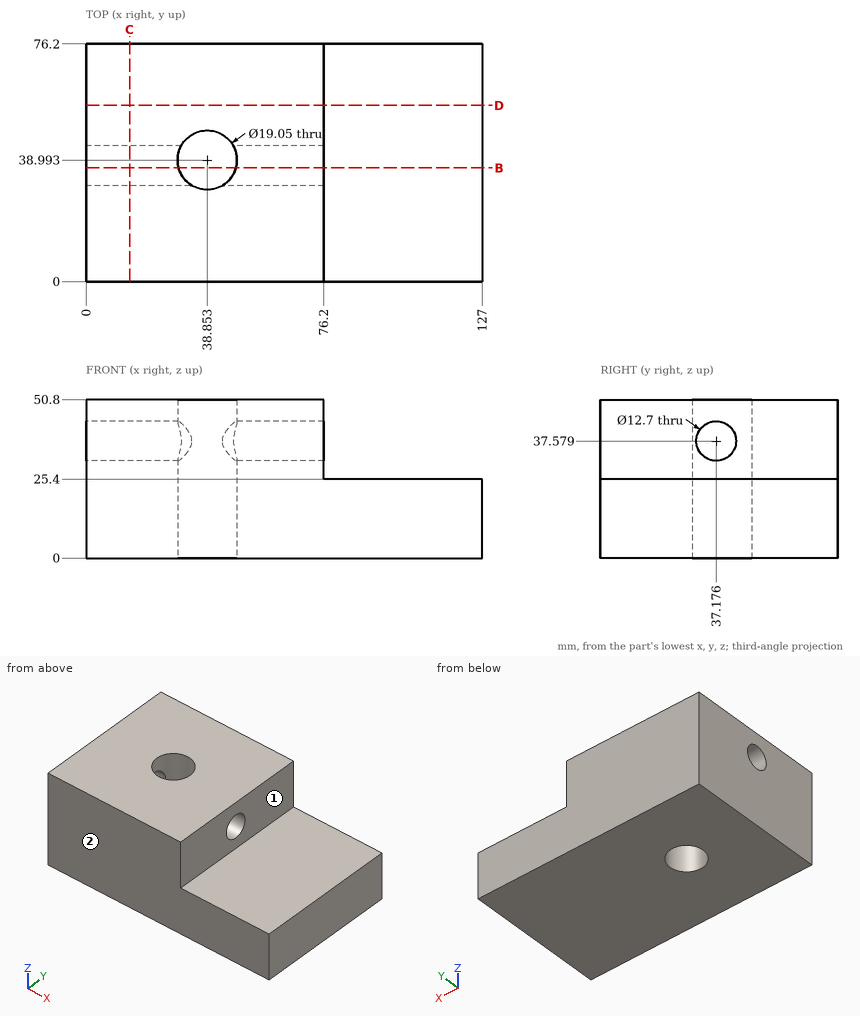
Check sheet for the drawn part. Datum: minimum x, y, z corner. Units: mm. A direction names the side the tool comes from. Coordinates: 2 decimals unless noted, no trailing zeros. Loops run counter-clockwise (first coordinate to the right, second up) from the corner with the lowest first, then second, coordinate; pieces in that order, holes last. Notation, with made-up numbers: (40.5, 66.5) -> (94.5, 66.5) arc R22 cw to (94.5, 80.5) -> close; hole circle Ø2 at (7, -28.75). An arc over 180 degrees is marked (long way). Answer in a Markdown table with one row per item.
1) Section check B-B (y = 36.5). Record the cut outline in (x, z) (1 decimal).
The answers:
| item | result |
|---|---|
| outline | (0, 0) -> (29.7, 0) -> (29.7, 31.3) -> (0, 31.3) -> close; (0, 43.9) -> (29.7, 43.9) -> (29.7, 50.8) -> (0, 50.8) -> close; (48, 0) -> (127, 0) -> (127, 25.4) -> (76.2, 25.4) -> (76.2, 31.3) -> (48, 31.3) -> close; (48, 43.9) -> (76.2, 43.9) -> (76.2, 50.8) -> (48, 50.8) -> close |
2) Section check D-D (y = 56.5). Record the cut outline in (x, z).
The answers:
| item | result |
|---|---|
| outline | (0, 0) -> (127, 0) -> (127, 25.4) -> (76.2, 25.4) -> (76.2, 50.8) -> (0, 50.8) -> close |
3) Depth check by flat-ended pin: P1, Ø10, axis at y = 37.18, z = 37.58, coming from the -X side; P2, Ø20.5, axis at y = 37.18, z = 37.58, coming from the +X side. Enter the tip coordinate at first touch or a pass-through.
The answers:
| item | result |
|---|---|
| P1 | passes through |
| P2 | stops at x = 76.2 |
4) Access from +Z, -Z, +X, -X, +Y, -Y to the whole of each face (thin tool, end or side, straight path). Record for the marked faces 1 and 2.
The answers:
| item | result |
|---|---|
| face 1 | +Z, +X, +Y, -Y |
| face 2 | +Z, -Z, +X, -X, -Y |
5) Scan lines: line 1 along Y through (x, z) = (16.5, 37); line 2 along X through (y, z) = (31.5, 18) (1 decimal); line 3 along X through (y, z) = (60, 46.5). Record each from-to range of solid material in increasing order. Write a range as from..to.
The answers:
| item | result |
|---|---|
| line 1 | y = 0..30.85, 43.5..76.2 |
| line 2 | x = 0..33, 44.7..127 |
| line 3 | x = 0..76.2 |
6) Section check C-C (x = 14). Record the cut outline in (y, z).
The answers:
| item | result |
|---|---|
| outline | (0, 0) -> (76.2, 0) -> (76.2, 50.8) -> (0, 50.8) -> close; hole circle Ø12.7 at (37.18, 37.58) |
